Can you work these out from the model? Positions are in its coordinate system, mm. Face numbers are marked on the shaded views. Give positions to 0.01 mm unless a question says otherwise; leave off trailing zeros. Loops run counter-clockwise (first coordinate to the right, second up) from the corner with the lowest first, then second, coordinate; pieces in that order, holes last. Notation, with made-up numbers: (-37.75, 81.25) -> (-18.75, 81.25) arc R33 ccw to (-18.75, 110.25) -> close; hole circle Ø3 at (5, 4). An arc over 180 degrees is marked (long way). Return JSON: item names as keys, results as strings. Group by question number.
Q1. Thinking about a two-plate mould opening in X: for the marked faces 1, 2, 3 and 4, which applies, pulls with the +X half, pulls with the -X half, needs draft (parallel to the pull), parting line crosses it, or undercut?
Q2. Suppose I cut it at C-C, the plane x = -13. Please give me the cut outline in (y, z), and give its area (3 significant figures).
Q3. Suppose I cut it at A-A, the plane z = 102. Please give me the cut outline in (x, y), and give its area (3 significant figures).
Q4. I need wall thicknesses on line 1 along X through (y, z) = (-583, 138); line 2 along Z through (x, y) = (-180, -327.5). Which ranges of each line are inside material? Lowest first, please. Write a range as [from, to].
Q5. Suppose I cut it at B-B, the plane y = 275. Please give me the cut outline in (x, z), and give its area (3 significant figures).
```python
from build123d import *

# Parameters (mm, degrees)
SKETCH2_W           = 600
SKETCH2_H           = 1500
BOSS_EXTRUDE1_DEPTH = 10
SKETCH5_W           = 10
SKETCH5_H           = 1500
EXTRUDE_THIN2_DEPTH = 200


with BuildPart() as part:
    # Sketch2 → Boss-Extrude1 (new body)
    with BuildSketch(Plane.XY):
        Rectangle(SKETCH2_W, SKETCH2_H)
    extrude(amount=BOSS_EXTRUDE1_DEPTH)

    # Sketch5 → Extrude-Thin2 (add)
    with BuildSketch(Plane(origin=(0, 0, 0), x_dir=(-1, 0, 0), z_dir=(0, 0, -1))):
        with Locations((-295, 0)):
            Rectangle(SKETCH5_W, SKETCH5_H)
        with Locations((295, 0)):
            Rectangle(SKETCH5_W, SKETCH5_H)
    extrude(amount=-EXTRUDE_THIN2_DEPTH)


solid = part.part
```
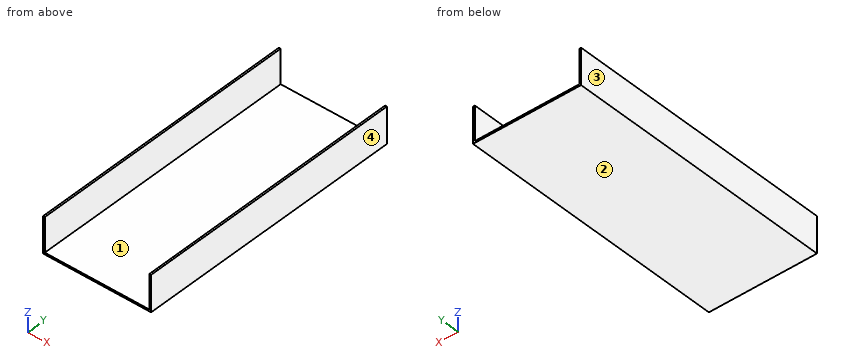
Ans:
{
 "1": {"face 1": "undercut", "face 2": "needs draft", "face 3": "pulls with the -X half", "face 4": "pulls with the +X half"},
 "2": {"outline": "(-750, 0) -> (750, 0) -> (750, 10) -> (-750, 10) -> close", "area": "15,000 mm^2"},
 "3": {"outline": "(-300, -750) -> (-290, -750) -> (-290, 750) -> (-300, 750) -> close; (290, -750) -> (300, -750) -> (300, 750) -> (290, 750) -> close", "area": "30,000 mm^2"},
 "4": {"line 1": "x = [-300, -290], [290, 300]", "line 2": "z = [0, 10]"},
 "5": {"outline": "(-300, 0) -> (300, 0) -> (300, 200) -> (290, 200) -> (290, 10) -> (-290, 10) -> (-290, 200) -> (-300, 200) -> close", "area": "9,800 mm^2"}
}
